Build history of the part. All positions in model axes, mm. Round coordinates to 2 decimals unless told otherwise and drop trailing zeros. Order: outer loops, then holes, each group sorted by start corner. A loop starts at its lowest first (then second) coordinate and runs counter-clockwise, first axis right, second up. Notation, with made-up numbers: (-9.75, 41) -> (42.25, 41) arc R15 cw to (42.25, 61) -> close; hole circle Ø11 at (-2.75, 40). An arc over 180 degrees is marked (long way). Use a Markdown table: item, result. Add a question column.
Item 1: Pin check, flat tips, straight feed: pin 1 (1 mm diameter, centred on x = -32.5, y = 0.5, fed in from -Z); pin 2 (1 mm diameter, centred on x = -14, y = 1, fed in from +Z); pin 3 (1 mm diameter, centred on y = 1.5, z = -2.5, fed in from +X). Stop position of each tip, or through.
Item 2: Probe L1, parallel to Z at x = 0, y = 0.95; L2, parallel to Z at x = -42, y = 0.3; L3, parallel to X at y = 0.9, z = 0.75. List the from-to ranges inside material, lowest first.
Item 3: Slice it at A-A, the plane x = 0. Give the cut face in (y, z).
Item 4: Two-plate mould, pull along Z, no slides. Class faces 1 (the face through (0, 1, 2)), 2 (the face through (-0.78, 0.99, -4.94)), 3 (the face through (0.789, 0.986, 4.937)): released by +Z, released by -Z, zero draft, split by the parting line, or undercut.
from build123d import *

# Parameters (mm, degrees)
ESQUISSE2_R        = 2
BOSS_EXTRU_1_DEPTH = 2


with BuildPart() as part:
    # Esquisse2 → Boss.-Extru.1 (new body)
    with BuildSketch(Plane(origin=(0, 0, 0), x_dir=(1, 0, 0), z_dir=(0, 1, 0))):
        with BuildLine():
            Line((5, 0), (76.2, 0))
            add(Edge.make_bspline(
                [(76.2, 0), (50.48496799, 16.589800369), (27.351766227, 10.012035882), (4.69008689, 1.732941131)],
                knots=[0.538892618, 0.538892618, 0.538892618, 0.538892618, 1, 1, 1, 1], degree=3))
            ThreePointArc((4.69008689, 1.732941131), (-0.880217459, 4.921911948), (-5, 0))
            Line((-5, 0), (-76.2, 0))
            add(Edge.make_bspline(
                [(-76.2, 0), (-51.013872042, -17.583290738), (-27.945849526, -10.334640761), (-4.686924988, -1.741474708)],
                knots=[0, 0, 0, 0, 0.475147649, 0.475147649, 0.475147649, 0.475147649], degree=3))
            ThreePointArc((-4.686924988, -1.741474708), (0.884696293, -4.921108866), (5, 0))
        make_face()
        Circle(ESQUISSE2_R, mode=Mode.SUBTRACT)
    extrude(amount=BOSS_EXTRU_1_DEPTH)


solid = part.part
Check sheet entries:
| question | item | result |
|---|---|---|
| 1 | pin 1 | z = 0 |
| 1 | pin 2 | z = 5.22 |
| 1 | pin 3 | x = 72.92 |
| 2 | L1 | -5 to -2, 2 to 5 |
| 2 | L2 | 0 to 10.78 |
| 2 | L3 | -75.1 to -1.85, 1.85 to 4.94 |
| 3 | outline | (0, -5) -> (2, -5) -> (2, -2) -> (0, -2) -> close; (0, 2) -> (2, 2) -> (2, 5) -> (0, 5) -> close |
| 4 | face 1 | undercut |
| 4 | face 2 | released by -Z |
| 4 | face 3 | released by +Z |
